```python
from build123d import *

# Parameters (mm, degrees)
BOSS_EXTRUDE1_DEPTH = 22.5
SKETCH2_R           = 1.5
CUT_EXTRUDE1_DEPTH  = 5
FILLET1_R           = 2
SKETCH4_W           = 55
SKETCH4_H           = 25
CUT_EXTRUDE3_DEPTH  = 10
SKETCH5_W           = 5
SKETCH5_H           = 5
CUT_EXTRUDE4_DEPTH  = 10
SKETCH6_W           = 60
SKETCH6_H           = 45
CUT_EXTRUDE5_DEPTH  = 10
FILLET2_R           = 10


with BuildPart() as part:
    # Sketch1 → Boss-Extrude1 (new, symmetric)
    with BuildSketch(Plane(origin=(0, 0, 0), x_dir=(1, 0, 0), z_dir=(0, 1, 0))):
        Polygon((-115, 0), (-85, 50), (85, 50), (115, 0), (108, 0), (81.6, 44), (-81.6, 44), (-108, 0), align=None)
    extrude(amount=BOSS_EXTRUDE1_DEPTH, both=True)

    # Sketch2 → Cut-Extrude1 (cut)
    with BuildSketch(Plane(origin=(0, 22.5, 0), x_dir=(1, 0, 0), z_dir=(0, 1, 0))):
        with Locations(Location((-103.701428863, 13, 0), (0, 0, 270))):
            Circle(SKETCH2_R)
        with Locations(Location((-77, 47, 0), (0, 0, 270))):
            Circle(SKETCH2_R)
        with Locations(Location((-7, 47, 0), (0, 0, 270))):
            Circle(SKETCH2_R)
        with Locations(Location((7, 47, 0), (0, 0, 90))):
            Circle(SKETCH2_R)
        with Locations(Location((77, 47, 0), (0, 0, 90))):
            Circle(SKETCH2_R)
        with Locations(Location((103.701428863, 13, 0), (0, 0, 90))):
            Circle(SKETCH2_R)
    extrude(amount=-CUT_EXTRUDE1_DEPTH, mode=Mode.SUBTRACT)

    # Fillet1
    fillet1_edges = [part.edges().sort_by_distance(p)[0] for p in [
        (-85, 0, -50),
        (85, 0, -50),
    ]]
    fillet(fillet1_edges, radius=FILLET1_R)

    # Sketch4 → Cut-Extrude3 (cut)
    with BuildSketch(Plane(origin=(84.558823529, 0, -50.735294118), x_dir=(-0.5144957554275265, 0, -0.8574929257125443), z_dir=(0.8574929257125443, 0, -0.5144957554275265))):
        with Locations((-31.667011874, -10)):
            Rectangle(SKETCH4_W, SKETCH4_H)
    extrude(amount=-CUT_EXTRUDE3_DEPTH, mode=Mode.SUBTRACT)

    # Sketch5 → Cut-Extrude4 (cut)
    with BuildSketch(Plane(origin=(-79.411764706, 0, -47.647058824), x_dir=(0.5144957554275261, 0, -0.8574929257125445), z_dir=(0.8574929257125444, 0, 0.514495755427526))):
        with Locations((-56.667011874, -20)):
            Rectangle(SKETCH5_W, SKETCH5_H)
    extrude(amount=-CUT_EXTRUDE4_DEPTH, mode=Mode.SUBTRACT)

    # Sketch6 → Cut-Extrude5 (cut)
    with BuildSketch(Plane(origin=(-79.411764706, 0, -47.647058824), x_dir=(0.5144957554275261, 0, -0.8574929257125445), z_dir=(0.8574929257125444, 0, 0.514495755427526))):
        with Locations((-34.253164912, 0)):
            Rectangle(SKETCH6_W, SKETCH6_H)
    extrude(amount=-CUT_EXTRUDE5_DEPTH, mode=Mode.SUBTRACT)

    # Fillet2
    fillet2_edges = [part.edges().sort_by_distance(p)[0] for p in [
        (81.6, 12.5, -44),
    ]]
    fillet(fillet2_edges, radius=FILLET2_R)


solid = part.part
```
Work out the finished part from the listing and answer in its coordinate system (mm). A direction names the side the tool comes from. Round coordinates to 2 decimals unless told otherwise and drop trailing zeros. Loops run counter-clockwise (first coordinate to the right, second up) from the corner with the lowest first, then second, coordinate; pieces in that order, holes last. Notation, with made-up numbers: M 40.25,6.5 L 98.25,6.5 A19 ccw 98.25,29.5 Z; hole C 80,32.25 d9. An arc over 180 degrees is marked long. Use CSV: the item, a comma, the result in double quotes.
Q1. Each of these flat-tipped pins is pushed along its axis until it touches: pin 1 (1.5 mm diameter, centred on x = 62, y = 3, fed in from +Z); pin 2 (1.5 mm diameter, centred on x = 7, z = -47, fed in from +Y); pin 3 (17.5 mm diameter, centred on x = 101, z = -23, fed in from -Y). Where does it stop, or does it pass through?
Determined:
pin 1,"z = -44"
pin 2,"y = 17.5"
pin 3,"y = 2.5"
Q2. Section C-C, the plane z = -3 is taken. Determine the outline of the cut face in (x, y).
Determined:
outline,"M 106.2,2.5 L 113.2,2.5 L 113.2,22.5 L 106.2,22.5 Z"
Q3. Section A-A, the plane y = -18 is taken. Determine the outline of the cut face in (x, z), then the cut area to 3 significant figures.
Determined:
outline,"M -86.75,-47.09 L -85.58,-49.03 A2 ccw -83.87,-50 L 83.87,-50 A2 ccw 85.58,-49.03 L 86.7,-47.16 L 80,-43.14 A10 cw 75.94,-44 L -81.6,-44 Z"
area,"1,020 mm2"
Q4. Section B-B, the plane x = 46 is taken. Determine the outline of the cut face in (y, z).
Determined:
outline,"M -22.5,-50 L 22.5,-50 L 22.5,-44 L -22.5,-44 Z"
Q5. Consider L1, parallel to X at y = 18.8, z = -47; L2, parallel to Y at x = 91.5, z = -35.5; L3, parallel to X at y = 20, z = -13. Determine where each line is inside the solid, lowest interval first.
Determined:
L1,"-86.6 to -78.5, -75.5 to -8.5, -5.5 to 5.5, 8.5 to 75.5, 78.5 to 86.8"
L2,"2.5 to 22.5"
L3,"100.2 to 102.2, 105.2 to 107.2"
Q6. A tool of negligible diameter and unlimited length cuts with its end or side. For faces 1 (the flat face through (83.4, -10.17, -45.18)), 2 (the flat face through (-2, 0, -44)), 3 (the flat face through (-1, 0, -50)), from which of +Z, -Z, +X, -X, +Y, -Y can it reach the whole face along a straight path? Write none if from no direction.
Determined:
face 1,"+Z, +X, -Y"
face 2,"+Z, -X, +Y, -Y"
face 3,"-Z, +X, -X, +Y, -Y"
